Part print with two shaded views. Sizes in mm from the minimum x, y, z corner. A direction names the side the tool comes from. Coordinates: 2 decimals unless noted, no trailing zeros. Loops run counter-clockwise (first coordinate to the right, second up) from the corner with the lowest first, then second, coordinate; pieces in that order, holes last. Notation, with made-up numbers: M -9,6 L 33,6 A19 ccw 33,31 Z; hole C 48,-4 d7. An arc over 180 degrees is marked long. Write item = value, one per line. Start each with the question number.
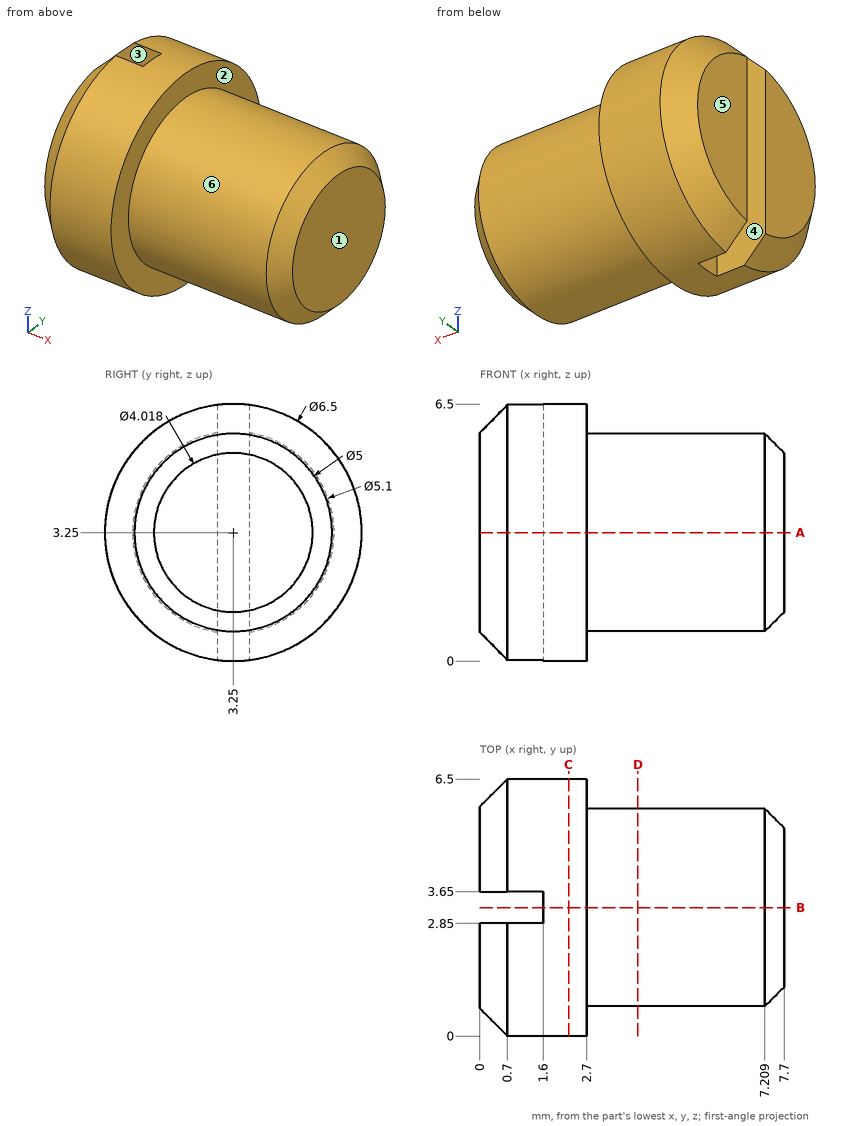
Item 1: Cut at A-A (z = 3.25). Give the cut face in (x, y).
Item 2: Cut at B-B (y = 3.25). Give the cut face in (x, z), plus the area to 3 significant figures.
Item 3: Pull direction Y, two halves, no side cores. Call the marked faces 4, 5 and 6: +Y half, -Y half, draft (parallel to the pull), parting line (faces both ways), or undercut.
Item 4: Pin check, flat tips, straight feed: pin 1 Ø0.8 at (x, z) = (1, 3.5) entering from -Y; pin 2 Ø1.5 at (x, y) = (3, 0.5) entering from -Z; pin 3 Ø1.8 at (x, z) = (0.5, 4.5) entering from +Y; pin 4 Ø1 at (x, z) = (3.5, 6) entering from -Y. Stop position of each tip, or through.
Item 5: Cut at C-C (x = 2.25). Give the cut face in (y, z).
Item 6: Probe L1, parallel to Y at x = 1.5, z = 4.5; L2, parallel to X at y = 3.5, z = 3.25; L3, parallel to Z at x = 3.5, y = 5.5. List the from-to ranges inside material, lowest first.
Item 7: 3-axis set-ups, long thin cutter, end or side, ignore diameter. For the marked faces 1, 2 and 3: which of +Z, -Z, +X, -X, +Y, -Y reach the whole face in a straight line?
Item 8: Cut at D-D (x = 4). Give the cut face in (y, z), plus the area to 3 significant figures.
Reported:
q1.outline = M 0,0.7 L 0.7,0 L 2.7,0 L 2.7,0.75 L 7.21,0.75 L 7.7,1.24 L 7.7,5.26 L 7.21,5.75 L 2.7,5.75 L 2.7,6.5 L 0.7,6.5 L 0,5.8 L 0,3.65 L 1.6,3.65 L 1.6,2.85 L 0,2.85 Z
q2.outline = M 1.6,0 L 2.7,0 L 2.7,0.75 L 7.21,0.75 L 7.7,1.24 L 7.7,5.26 L 7.21,5.75 L 2.7,5.75 L 2.7,6.5 L 1.6,6.5 Z
q2.area = 31.9 mm^2
q3.face_4 = undercut
q3.face_5 = draft
q3.face_6 = parting line
q4.pin_1 = 0
q4.pin_2 = 0.74
q4.pin_3 = 6.48
q4.pin_4 = 2.16
q5.outline = C 3.25,3.25 d6.5
q6.L1 = 0.25 to 2.85, 3.65 to 6.25
q6.L2 = 1.6 to 7.7
q6.L3 = 2.16 to 4.34
q7.face_1 = +Z, -Z, +X, +Y, -Y
q7.face_2 = +X
q7.face_3 = +Z, -Z, -X
q8.outline = C 3.25,3.25 d5
q8.area = 19.6 mm^2
